The listing builds one solid part. Answer for the finished solid, in the listing's coordinates (mm). Round coordinates to 2 decimals unless told otherwise and drop trailing zeros. Write each loop counter-clockwise with the first axis right and the second up, starting at its lowest first coordinate (ties: lowest second). Pieces come first, ordered by that corner, then holes. Notation, with made-up numbers: M 52.25,83.5 L 105.25,83.5 A12 cw 105.25,87.5 Z; hole C 29.5,65.5 d5. An arc over 180 degrees is marked long. One line per item, written item: value. Start each with the question number.
(1) Consider probe 1 along Y at (x, z) = (140.25, 3.75); probe 2 along Y at (x, z) = (-271, 3.25); probe 3 along Y at (x, z) = (-200.5, 4). Determine where each line is inside the solid, lowest interval first.
(2) Given P1, Ø3, axis at x = -140.25, y = 451.5, coming from the -Z side, flat-ended and moving along its own axis, determine where the tip first touches the part or whether it passes through.
(3) For a pull along X with two mould halves and no side action, classify faces 1 (the flat face through (-4, 234, 9)), 2 (the cylindrical face through (-197.245, 435.787, 4.563)) as released by +X, released by -X, zero draft, split by the parting line, or undercut.
(4) Section A-A (x = -200.5) is taken. Determine the outline of the cut face in (y, z), plus the area to 3 significant figures.
```python
from build123d import *

# Parameters (mm, degrees)
SKETCH_1_W               = 561
SKETCH_1_H               = 461
SKETCH_1_R               = 2.5
EXTRUDE_1_DEPTH          = 9
CUT_EXTRUDE_1_DEPTH      = 540.705706844
CUT_EXTRUDE_1_DEPTH_BACK = 540.705706844
SKETCH_2_R               = 25


with BuildPart() as part:
    # 草图1 → 凸台-拉伸1 (new body)
    with BuildSketch(Plane.XY):
        with Locations((0, 230.5)):
            Rectangle(SKETCH_1_W, SKETCH_1_H)
        with Locations((-140.25, 451.5)):
            Circle(SKETCH_1_R, mode=Mode.SUBTRACT)
        with Locations((-271, 345.75)):
            Circle(SKETCH_1_R, mode=Mode.SUBTRACT)
        with Locations(Location((271, 345.75, 0), (0, 0, 180))):
            Circle(SKETCH_1_R, mode=Mode.SUBTRACT)
        with Locations(Location((140.25, 451.5, 0), (0, 0, 180))):
            Circle(SKETCH_1_R, mode=Mode.SUBTRACT)
        with Locations((271, 115.25)):
            Circle(SKETCH_1_R, mode=Mode.SUBTRACT)
        with Locations((140.25, 9.5)):
            Circle(SKETCH_1_R, mode=Mode.SUBTRACT)
        with Locations(Location((-271, 115.25, 0), (0, 0, 180))):
            Circle(SKETCH_1_R, mode=Mode.SUBTRACT)
        with Locations(Location((-140.25, 9.5, 0), (0, 0, 180))):
            Circle(SKETCH_1_R, mode=Mode.SUBTRACT)
    extrude(amount=EXTRUDE_1_DEPTH)

    # 草图2 → 切除-拉伸1 (cut, two sides: drawn at the far end of the back side and taken through both)
    with BuildSketch(Plane(origin=(0, 0, 0), x_dir=(-1, 0, 0), z_dir=(0, 0, -1)).offset(-CUT_EXTRUDE_1_DEPTH_BACK)):
        with Locations((200.5, 411)):
            Circle(SKETCH_2_R)
    extrude(amount=CUT_EXTRUDE_1_DEPTH + CUT_EXTRUDE_1_DEPTH_BACK, mode=Mode.SUBTRACT)


solid = part.part
```
Recorded:
1. probe 1: y = 0 to 7, 12 to 449, 454 to 461
1. probe 2: y = 0 to 112.75, 117.75 to 343.25, 348.25 to 461
1. probe 3: y = 0 to 386, 436 to 461
2. P1: passes through
3. face 1: zero draft
3. face 2: undercut
4. outline: M 0,0 L 386,0 L 386,9 L 0,9 Z; M 436,0 L 461,0 L 461,9 L 436,9 Z
4. area: 3,700 mm2
